```python
from build123d import *

# Parameters (mm, degrees)
BOSS_EXTRUDE1_DEPTH = 2
BOSS_EXTRUDE2_DEPTH = 2


with BuildPart() as part:
    # Sketch1 → Boss-Extrude1 (new body)
    with BuildSketch(Plane.XY):
        with BuildLine():
            Line((0, 0), (0, 6))
            ThreePointArc((0, 6), (-4.242640687, 4.242640687), (-6, 0))
            Line((-6, 0), (0, 0))
        make_face()
    extrude(amount=BOSS_EXTRUDE1_DEPTH)

    # Sketch2 → Boss-Extrude2 (add)
    with BuildSketch(Plane.XZ):
        with BuildLine():
            ThreePointArc((-2.983237378, 3.741602043), (-3.256022499, 2.733272353), (-3.999966142, 2))
            Line((-3.999966142, 2), (-1.000033858, 2))
            ThreePointArc((-1.000033858, 2), (-2.319710429, 2.497214459), (-2.983237378, 3.741602043))
        make_face()
    extrude(amount=-BOSS_EXTRUDE2_DEPTH)


solid = part.part
```
Here's how the part is built. I have some questions about the finished solid (model axes, mm). A direction names the side the tool comes from. Coordinates: 2 decimals unless noted, no trailing zeros. Order: outer loops, then holes, each group sorted by start corner. A loop starts at its lowest first (then second) coordinate and runs counter-clockwise, first axis right, second up. Notation, with made-up numbers: M 24,78 L 39,78 A21 ccw 39,86 Z; hole C 10.25,79.25 d10. An arc over 180 degrees is marked long. Answer as a JSON object with one key per item and string values. Group by question number.
(1) Suppose I cut it at C-C, the plane z = 1.75. Please give me the cut outline in (x, y), then the cut area to 3 significant figures.
(2) Suppose I cut it at B-B, the plane x = -0.75. Please give me the cut outline in (y, z), then the cut area to 3 significant figures.
(3) Suppose I cut it at A-A, the plane y = 0.75. Please give me the cut outline in (x, z).
(4) I need wall thicknesses on probe 1 along Z at (x, y) = (-0.25, 1.5); probe 2 along X at (y, z) = (5.25, 0.5); probe 3 along X at (y, z) = (0.5, 2.85). Which ranges of each line are inside material? Lowest first, please.
(5) For pin 1 (1 mm diameter, centred on y = 3, z = 1, fed in from -X); pin 2 (1.5 mm diameter, centred on x = -3, z = 2.5, fed in from +Y), each with a flat end and sliding along its axis, tell me the tip position at first contact or that it passes through.
(6) Which directions (+Z, -Z, +X, -X, +Y, -Y) give clear straight access to the entire face, cutting with the end or side of a thin tool? Please do faces 1 (the face through (-3.249, 0.986, 2.746)), 2 (the face through (-2.8, 2, 2.4)).
(7) Suppose I cut it at D-D, the plane x = -4.25. Please give me the cut outline in (y, z), then the cut area to 3 significant figures.
Values found:
{
 "1": {"outline": "M -6,0 L 0,0 L 0,6 A6 ccw Z", "area": "28.3 mm^2"},
 "2": {"outline": "M 0,0 L 5.95,0 L 5.95,2 L 0,2 Z", "area": "11.9 mm^2"},
 "3": {"outline": "M -5.95,0 L 0,0 L 0,2 L -1,2 A2 cw -2.98,3.74 A2 cw -4,2 L -5.95,2 Z"},
 "4": {"probe 1": "z = 0 to 2", "probe 2": "x = -2.9 to 0", "probe 3": "x = -3.19 to -2.64"},
 "5": {"pin 1": "stops at x = -5.45", "pin 2": "stops at y = 5.48"},
 "6": {"face 1": "+Z, -X, +Y, -Y", "face 2": "+Z, +X, -X, +Y"},
 "7": {"outline": "M 0,0 L 4.24,0 L 4.24,2 L 0,2 Z", "area": "8.47 mm^2"}
}
